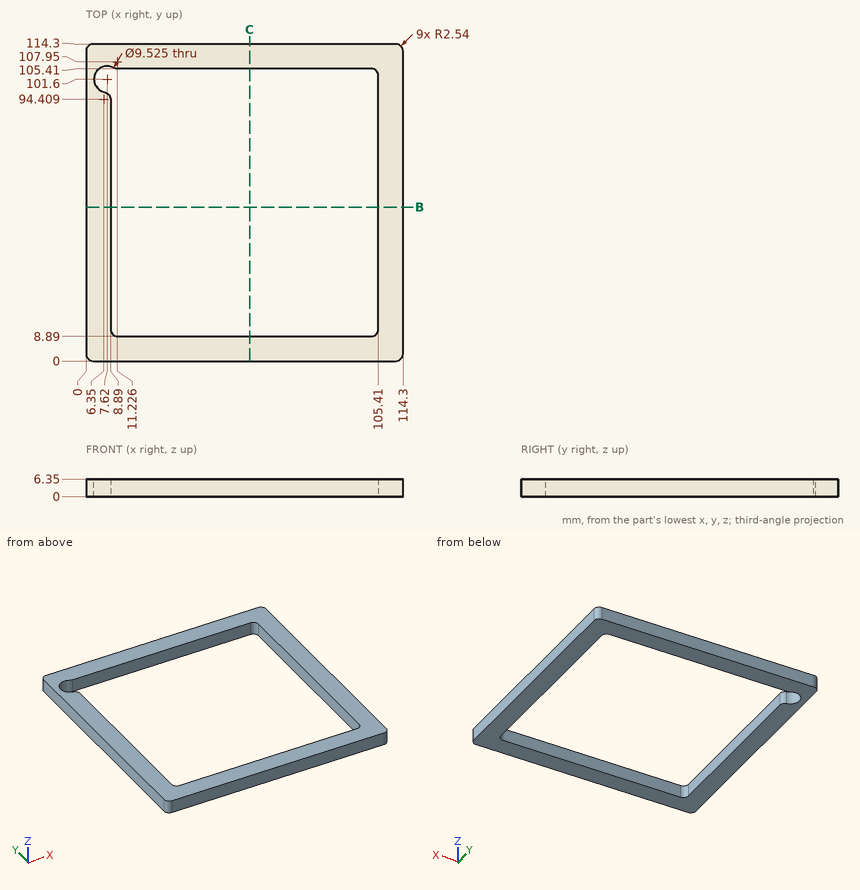
The drawing under review shows one solid part. Ordinate dimensions are in mm from its lowest x, y, z. Coordinates: 2 decimals unless noted, no trailing zeros. Order: outer loops, then holes, each group sorted by start corner. A loop starts at its lowest first (then second) coordinate and runs counter-clockwise, first axis right, second up. Notation, with made-up numbers: (51, -26.75) -> (92, -26.75) arc R19 cw to (92, -7.75) -> close; hole circle Ø6 at (75.25, -21). An arc over 180 degrees is marked (long way). One line per item, written item: value.
1) We need section B-B, the plane y = 55.5. Give the boundary of the cut face in (x, z).
Output values:
outline: (0, 0) -> (8.89, 0) -> (8.89, 6.35) -> (0, 6.35) -> close; (105.41, 0) -> (114.3, 0) -> (114.3, 6.35) -> (105.41, 6.35) -> close
2) To check wall thickness, follow probe 1 along Y at (x, z) = (69, 3.5); probe 2 along X at (y, z) = (101.6, 3.25). State the ranges of each line that lie inside material, in increasing order. Write a range as [from, to].
Output values:
probe 1: y = [0, 8.89], [105.41, 114.3]
probe 2: x = [0, 2.86], [105.41, 114.3]
